from build123d import *

# Parameters (mm, degrees)
F1_DEPTH       = 45
F2_W           = 45
F2_H           = 65
F3_DEPTH       = 8
F4_R           = 9.99999
F6_R           = 8
F7_R           = 3
F9_D           = 7
F9_CSINK_D     = 10
F9_CSINK_ANGLE = 90


# Not quite as in the source:
# - two fillets or chamfers of one size are made in one step
# - a fillet or chamfer is up to 0.001 mm smaller than in the source, because OpenCascade refuses the exact size


with BuildPart() as f1:
    # F0 (on Top) → F1 (new body)
    with BuildSketch(Plane.XY):
        Polygon((8, 105), (0, 105), (0, 0), (36, 0), (36, 60), (28, 60), (28, 10), (8, 10), align=None)
    extrude(amount=F1_DEPTH)

    # F2 (on Right) → F3 (join, through all)
    with BuildSketch(Plane.YZ):
        with Locations((82.5, 32.5)):
            Rectangle(F2_W, F2_H)
    extrude(amount=F3_DEPTH)

    # F4 (radius 10 in the source; OpenCascade refuses exactly that, so slightly less here)
    f4_edges = [f1.edges().sort_by_distance(p)[0] for p in [
        (4, 60, 45),
        (4, 105, 0),
        (4, 105, 65),
        (4, 60, 65),
        (32, 60, 45),
        (32, 60, 0),
        (36, 0, 22.5),
    ]]
    fillet(f4_edges, radius=F4_R)

    # F6
    f6_edges = [f1.edges().sort_by_distance(p)[0] for p in [
        (8, 10, 22.5),
        (28, 10, 22.5),
    ]]
    fillet(f6_edges, radius=F6_R)

    # F7
    f7_edges = [f1.edges().sort_by_distance(p)[0] for p in [
        (36, 60, 22.5),
        (36, 57.071071, 2.928929),
        (36, 57.071071, 42.071071),
        (36, 30, 0),
        (36, 30, 45),
        (36, 9.99999, 22.5),
        (8, 56.500005, 0),
        (8, 18, 22.5),
        (8, 102.071071, 2.928929),
        (8, 34.000005, 45),
        (8, 105, 32.5),
        (8, 57.071071, 47.928929),
        (8, 102.071071, 62.071071),
        (8, 60, 55),
        (8, 82.5, 65),
        (8, 62.928929, 62.071071),
        (10.343146, 12.343146, 0),
        (18, 10, 0),
        (25.656854, 12.343146, 0),
        (13.000005, 0, 0),
        (28, 34.000005, 0),
        (33.071071, 2.928929, 0),
        (10.343146, 12.343146, 45),
        (18, 10, 45),
        (25.656854, 12.343146, 45),
        (13.000005, 0, 45),
        (28, 34.000005, 45),
        (33.071071, 2.928929, 45),
        (28, 57.071071, 2.928929),
        (28, 60, 22.5),
        (28, 57.071071, 42.071071),
    ]]
    fillet(f7_edges, radius=F7_R)

    # F9 (through all)
    with Locations(Plane.YZ.offset(8)):
        with Locations((83, 51.8898591027), (83, 16.8898591027)):
            CounterSinkHole(F9_D / 2, F9_CSINK_D / 2, counter_sink_angle=F9_CSINK_ANGLE)


solid = f1.part
Model file for the job. Use its own axes, mm. A direction names the side the tool comes from. Coordinates: 2 decimals unless noted, no trailing zeros. Order: outer loops, then holes, each group sorted by start corner. A loop starts at its lowest first (then second) coordinate and runs counter-clockwise, first axis right, second up. Notation, with made-up numbers: (-10.75, -29) -> (18.25, -29) arc R37 cw to (18.25, 7) -> close; hole circle Ø8 at (-11, -3). An arc over 180 degrees is marked (long way). Return JSON: item names as keys, results as strings. Group by question number.
Item 1: Tool access for faces 5 (the cylindrical face through (7.14, 33.78, 44.1)), 6 (the cylindrical face through (31.99, 56.99, 42.15)), 7 (the cylindrical face through (28.86, 59.1, 22.32)): list every direction of +Z, -Z, +X, -X, +Y, -Y with a clear straight run to the whole face (end or side of a thin tool).
Item 2: Pull direction Z, two halves, no side cores. Call faces 1 (the cylindrical face through (3.2, 79.66, 52.94)), 2 (the flat face through (3, 105, 32)), 3 (the cylindrical face through (7.14, 57.04, 0.9)), 4 (the cylindrical face through (2.54, 102.15, 61.99)): pulls with the +Z half, pulls with the -Z half, needs draft (parallel to the pull), parting line crosses it, or undercut.
Item 3: Saw through at A-A on y = 83. Write the cut outline in (x, z).
Item 4: Saw through at C-C on x = 18. Write the cut outline in (y, z), then the cut area to 3 significant figures.
Item 5: Saw through at B-B on z = 33. Write the cut outline in (x, y).
Item 6: Wall check: line 1 along Z through (x, y) = (4.75, 83); line 2 along X through (y, z) = (37.5, 16.5); line 3 along X through (y, z) = (16.5, 3). Give the ranges that are in metal, low to high. Write a range as [from, to].
Item 7: Flat gauge pins, fed straight in: P1, Ø1, axis at y = 80, z = 30.5, coming from the +X side; P2, Ø2, axis at x = 18.5, z = 22.5, coming from the +Y side; P3, Ø1, axis at x = 32.5, z = 27.5, coming from the +Y side. Where does each tip first touch, or does it go through?
Values found:
{
 "1": {"face 5": "+Z", "face 6": "+Z, +X, +Y", "face 7": "+Z, -Z, +Y"},
 "2": {"face 1": "undercut", "face 2": "needs draft", "face 3": "pulls with the -Z half", "face 4": "pulls with the +Z half"},
 "3": {"outline": "(0, 0) -> (5, 0) arc R3 ccw to (8, 3) -> (8, 11.89) -> (6.5, 13.39) -> (0, 13.39) -> close; (0, 20.39) -> (6.5, 20.39) -> (8, 21.89) -> (8, 46.89) -> (6.5, 48.39) -> (0, 48.39) -> close; (0, 55.39) -> (6.5, 55.39) -> (8, 56.89) -> (8, 62) arc R3 ccw to (5, 65) -> (0, 65) -> close"},
 "4": {"outline": "(0, 3) arc R3 ccw to (3, 0) -> (7, 0) arc R3 ccw to (10, 3) -> (10, 42) arc R3 ccw to (7, 45) -> (3, 45) arc R3 ccw to (0, 42) -> close", "area": "442 mm2"},
 "5": {"outline": "(0, 0) -> (26, 0) arc R10 ccw to (36, 10) -> (36, 57) arc R3 ccw to (33, 60) -> (31, 60) arc R3 ccw to (28, 57) -> (28, 18) arc R8 cw to (20, 10) -> (16, 10) arc R8 cw to (8, 18) -> (8, 102) arc R3 ccw to (5, 105) -> (0, 105) -> close"},
 "6": {"line 1": "z = [0, 13.39], [20.39, 48.39], [55.39, 65]", "line 2": "x = [0, 8], [28, 36]", "line 3": "x = [0, 8.14], [27.86, 36]"},
 "7": {"P1": "stops at x = 8", "P2": "stops at y = 10", "P3": "stops at y = 60"}
}
